Source: three-view drawing plus pictorial views. Frame: mm from the lowest corner of the part. A direction names the side the tool comes from. Round coordinates to 2 decimals unless told otherwise and drop trailing zeros. Order: outer loops, then holes, each group sorted by start corner. A loop starts at its lowest first (then second) coordinate and runs counter-clockwise, first axis right, second up. Notation, with made-up numbers: (29, -6) -> (36, -6) arc R28 cw to (36, 13) -> close; hole circle Ø11 at (14, -40). An arc over 180 degrees is marked (long way). Use a Markdown table: item, result.
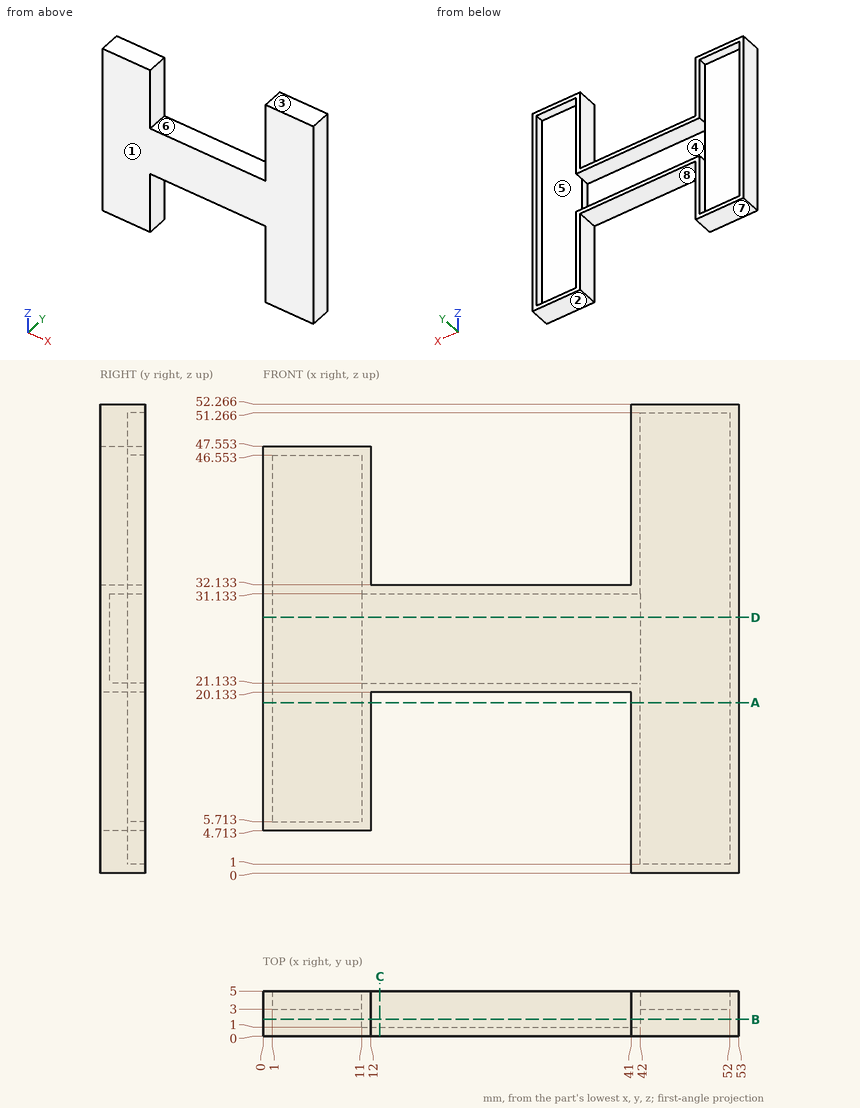
1) Pin query (flat end, axial travel): pin 1 Ø2.5 at (x, y) = (33, 3) entering from +Z; pin 2 Ø1.6 at (y, z) = (2.5, 26) entering from -X; pin 3 Ø2.5 at (x, y) = (7, 3.5) entering from +Z; pin 4 Ø1.5 at (x, y) = (32, 2) entering from -Z. Return the tip coordinate at first contact, or that it passes through.
Results found:
| item | result |
|---|---|
| pin 1 | stops at z = 32.13 |
| pin 2 | stops at x = 0 |
| pin 3 | stops at z = 47.55 |
| pin 4 | stops at z = 20.13 |
2) Cut plane C-C on x = 13. Return loops of the section in (y, z).
Results found:
| item | result |
|---|---|
| outline | (0, 20.13) -> (5, 20.13) -> (5, 21.13) -> (1, 21.13) -> (1, 31.13) -> (5, 31.13) -> (5, 32.13) -> (0, 32.13) -> close |
3) Set-up query: the marked faces 5, 6, 7 and 8. Return all of +Z, -Z, +X, -X, +Y, -Y with unobstructed straight access to the full face (end or side cutting, diameter ignored); none if empty.
Results found:
| item | result |
|---|---|
| face 5 | +Y |
| face 6 | +Z, +Y, -Y |
| face 7 | -Z, -X, +Y, -Y |
| face 8 | -Z, +Y, -Y |
4) Pull-direction query (Z, two-part tool) for the marked faces 1, 2, 3 and 4; classes: +Z half, -Z half, draft (parallel to the pull), parting line (faces both ways), or undercut.
Results found:
| item | result |
|---|---|
| face 1 | draft |
| face 2 | -Z half |
| face 3 | +Z half |
| face 4 | undercut |
5) Cut plane D-D on z = 28.5. Return loops of the section in (x, y), and give its area (3 significant figures).
Results found:
| item | result |
|---|---|
| outline | (0, 0) -> (53, 0) -> (53, 5) -> (52, 5) -> (52, 3) -> (42, 3) -> (42, 1) -> (11, 1) -> (11, 3) -> (1, 3) -> (1, 5) -> (0, 5) -> close |
| area | 101 mm² |
6) Line query: L1, parallel to X at y = 3.2, z = 8; L2, parallel to X at y = 2.3, z = 12.5; L3, parallel to Z at x = 19, y = 2.65. Output: solid intervals per line, ascending. Write a range as [from, to].
Results found:
| item | result |
|---|---|
| L1 | x = [0, 1], [11, 12], [41, 42], [52, 53] |
| L2 | x = [0, 12], [41, 53] |
| L3 | z = [20.13, 21.13], [31.13, 32.13] |
7) Cut plane B-B on y = 1.85. Return loops of the section in (x, z).
Results found:
| item | result |
|---|---|
| outline | (0, 4.71) -> (12, 4.71) -> (12, 20.13) -> (41, 20.13) -> (41, 0) -> (53, 0) -> (53, 52.27) -> (41, 52.27) -> (41, 32.13) -> (12, 32.13) -> (12, 47.55) -> (0, 47.55) -> close; hole (11, 21.13) -> (42, 21.13) -> (42, 31.13) -> (11, 31.13) -> close |
8) Cut plane A-A on z = 19. Return loops of the section in (x, y).
Results found:
| item | result |
|---|---|
| outline | (0, 0) -> (12, 0) -> (12, 5) -> (11, 5) -> (11, 3) -> (1, 3) -> (1, 5) -> (0, 5) -> close; (41, 0) -> (53, 0) -> (53, 5) -> (52, 5) -> (52, 3) -> (42, 3) -> (42, 5) -> (41, 5) -> close |
